Geometry check sheet. Reference: the model listing, model coordinates, mm. A direction names the side the tool comes from. Coordinates: 2 decimals unless noted, no trailing zeros. Loops run counter-clockwise (first coordinate to the right, second up) from the corner with the lowest first, then second, coordinate; pieces in that order, holes last.
Autodesk Inventor part; units mm, degrees
ref_plane "YZ Plane" through (0, 0, 0) normal (1, 0, 0) x (0, 1, 0)
ref_plane "XZ Plane" through (0, 0, 0) normal (0, 1, 0) x (-1, 0, 0)
ref_plane "XY Plane" through (0, 0, 0) normal (0, 0, 1) x (1, 0, 0)
sketch "スケッチ1" plane through (0, 0, 0) normal (0, 0, 1) x (1, 0, 0)
  line L0 (67.5, 17.5) -> (-67.5, 17.5) construction
  line L1 (-67.5, 17.5) -> (-67.5, -17.5) construction
  line L2 (-67.5, -17.5) -> (67.5, -17.5) construction
  line L3 (67.5, -17.5) -> (67.5, 17.5) construction
  line L4 (67.5, 17.5) -> (-67.5, -17.5) construction
  line L5 (-67.5, 17.5) -> (67.5, -17.5) construction
  circle A0 centre (-60, 35) radius 1.6 construction
  circle A1 centre (-70, 35) radius 1.6 construction
  line L6 (-77.5, 27.5) -> (-53, 27.5) construction
  line L7 (-53, 27.5) -> (-53, 42.5) construction
  line L8 (-53, 42.5) -> (-80, 42.5) construction
  line L9 (-77.5, 27.5) -> (-77.5, -27.5) construction
  line L10 (-77.5, -27.5) -> (-53, -27.5) construction
  line L11 (-53, -27.5) -> (-53, -42.5) construction
  line L12 (-53, -42.5) -> (-80, -42.5) construction
  circle A2 centre (-60, -35) radius 1.6 construction
  circle A3 centre (-70, -35) radius 1.6 construction
  circle A4 centre (-80, -35) radius 1.6 construction
  line L13 (124.2308, -31.7536) -> (484.5935, -392.1164)
  line L14 (484.5935, -392.1164) -> (488.7129, -553.575)
  line L15 (-80, 21.2868) -> (-468.838, -367.5512) construction
  line L16 (-468.838, -367.5512) -> (-479.4446, -356.9446)
  line L17 (-479.4446, -356.9446) -> (-90.6066, 31.8934) construction
  line L18 (-90.6066, 31.8934) -> (-80, 21.2868) construction
  line L19 (-80, 42.5) -> (-80, 5.3052) construction
  circle A5 centre (-92.3744, 19.519) radius 1.6 construction
  circle A6 centre (-102.981, 8.9124) radius 1.6 construction
  circle A7 centre (-113.5876, -1.6942) radius 1.6 construction
  line L20 (-92.3744, 19.519) -> (-113.5876, -1.6942) construction
  circle A8 centre (-437.941, -345.2067) radius 1.6
  circle A9 centre (-426.1402, -333.4059) radius 1.6
  line L21 (-388.4374, -772.2067) -> (-358.1265, -754.7067) construction
  line L22 (-358.1265, -754.7067) -> (-425.6265, -637.7933) construction
  line L23 (-455.9374, -655.2933) -> (-358.1265, -754.7067) construction
  line L24 (-388.4374, -772.2067) -> (-425.6265, -637.7933) construction
  line L25 (-455.9374, -655.2933) -> (-388.4374, -772.2067) construction
  line L26 (-425.6265, -637.7933) -> (-455.9374, -655.2933) construction
  line L27 (455.9374, -655.2933) -> (425.6265, -637.7933) construction
  line L28 (425.6265, -637.7933) -> (358.1265, -754.7067) construction
  line L29 (388.4374, -772.2067) -> (425.6265, -637.7933) construction
  line L30 (455.9374, -655.2933) -> (358.1265, -754.7067) construction
  line L31 (388.4374, -772.2067) -> (455.9374, -655.2933) construction
  line L32 (358.1265, -754.7067) -> (388.4374, -772.2067) construction
  line L33 (0, 0) -> (0, -263.4473) construction
  circle A10 centre (80, -35) radius 1.6 construction
  line L34 (67.5, 17.5) -> (67.5, -17.5) construction
  line L35 (77.5, 27.5) -> (53, 27.5) construction
  line L36 (77.5, 27.5) -> (77.5, -27.5) construction
  line L37 (77.5, -27.5) -> (53, -27.5) construction
  circle A11 centre (60, -35) radius 1.6 construction
  circle A12 centre (70, -35) radius 1.6 construction
  line L38 (53, -27.5) -> (53, -42.5) construction
  line L39 (53, -42.5) -> (80, -42.5) construction
  circle A13 centre (60, 35) radius 1.6 construction
  circle A14 centre (70, 35) radius 1.6 construction
  line L40 (80, 42.5) -> (80, 5.3052) construction
  line L41 (53, 42.5) -> (80, 42.5) construction
  line L42 (53, 27.5) -> (53, 42.5) construction
  line L43 (-392.0976, -785.867) -> (-404.3476, -764.6493)
  line L44 (-388.4374, -772.2067) -> (-358.1265, -754.7067) construction
  line L45 (-392.0976, -785.867) -> (-344.4662, -758.367)
  circle A15 centre (-336.7211, -756.782) radius 1.6
  circle A16 centre (-341.7211, -748.1218) radius 1.6
  line L46 (-343.7259, -729.6493) -> (-330.2259, -753.032)
  circle A17 centre (-346.7211, -739.4615) radius 1.6
  line L47 (-356.7162, -737.1493) -> (-343.7259, -729.6493)
  line L48 (-344.4662, -758.367) -> (-356.7162, -737.1493)
  circle A18 centre (-407.3428, -774.4615) radius 1.6
  circle A19 centre (-402.3428, -783.1218) radius 1.6
  line L49 (-404.3476, -764.6493) -> (-417.338, -772.1493)
  line L50 (-417.338, -772.1493) -> (-403.838, -795.532)
  line L51 (-403.838, -795.532) -> (-371.6264, -776.9346) construction
  line L52 (-425.6265, -637.7933) -> (-455.9374, -655.2933) construction
  line L53 (-409.7162, -645.3507) -> (-396.7259, -637.8507)
  circle A20 centre (-406.7211, -635.5385) radius 1.6
  line L54 (-455.9374, -655.2933) -> (-425.6265, -637.7933) construction
  circle A21 centre (-411.7211, -626.8782) radius 1.6
  line L55 (-469.5976, -651.633) -> (-421.9662, -624.133)
  line L56 (-421.9662, -624.133) -> (-409.7162, -645.3507)
  line L57 (-396.7259, -637.8507) -> (-410.2259, -614.468)
  circle A22 centre (-416.7211, -618.218) radius 1.6
  line L58 (-469.5976, -651.633) -> (-457.3476, -672.8507)
  circle A23 centre (-467.3428, -670.5385) radius 1.6
  circle A24 centre (-472.3428, -661.8782) radius 1.6
  line L59 (-483.838, -656.968) -> (-451.6264, -638.3706) construction
  line L60 (-470.338, -680.3507) -> (-483.838, -656.968)
  line L61 (-457.3476, -672.8507) -> (-470.338, -680.3507)
  line L62 (469.5976, -651.633) -> (457.3476, -672.8507)
  line L63 (455.9374, -655.2933) -> (425.6265, -637.7933) construction
  line L64 (469.5976, -651.633) -> (421.9662, -624.133)
  circle A25 centre (416.7211, -618.218) radius 1.6
  circle A26 centre (411.7211, -626.8782) radius 1.6
  line L65 (396.7259, -637.8507) -> (410.2259, -614.468)
  circle A27 centre (406.7211, -635.5385) radius 1.6
  line L66 (409.7162, -645.3507) -> (396.7259, -637.8507)
  line L67 (421.9662, -624.133) -> (409.7162, -645.3507)
  circle A28 centre (467.3428, -670.5385) radius 1.6
  circle A29 centre (472.3428, -661.8782) radius 1.6
  line L68 (457.3476, -672.8507) -> (470.338, -680.3507)
  line L69 (470.338, -680.3507) -> (483.838, -656.968)
  line L70 (483.838, -656.968) -> (451.6264, -638.3706) construction
  line L71 (358.1265, -754.7067) -> (388.4374, -772.2067) construction
  line L72 (356.7162, -737.1493) -> (343.7259, -729.6493)
  circle A30 centre (346.7211, -739.4615) radius 1.6
  line L73 (388.4374, -772.2067) -> (358.1265, -754.7067) construction
  circle A31 centre (341.7211, -748.1218) radius 1.6
  line L74 (392.0976, -785.867) -> (344.4662, -758.367)
  line L75 (344.4662, -758.367) -> (356.7162, -737.1493)
  line L76 (343.7259, -729.6493) -> (330.2259, -753.032)
  circle A32 centre (336.7211, -756.782) radius 1.6
  line L77 (392.0976, -785.867) -> (404.3476, -764.6493)
  circle A33 centre (407.3428, -774.4615) radius 1.6
  circle A34 centre (402.3428, -783.1218) radius 1.6
  line L78 (403.838, -795.532) -> (371.6264, -776.9346) construction
  line L79 (417.338, -772.1493) -> (403.838, -795.532)
  line L80 (404.3476, -764.6493) -> (417.338, -772.1493)
  line L81 (-483.838, -367.5512) -> (-468.838, -367.5512)
  line L82 (-468.838, -367.5512) -> (-468.838, -648.3077) construction
  line L83 (-468.838, -648.3077) -> (-483.838, -648.3077) construction
  line L84 (-483.838, -648.3077) -> (-483.838, -367.5512) construction
  line L85 (-283.2277, -604.4352) -> (-262.2277, -640.8083) construction
  line L86 (345.2492, -497.0108) -> (305.7786, -565.3759) construction
  line L87 (260.9224, -655.004) -> (-239.0776, -655.004) construction
  line L88 (-239.0776, -655.004) -> (-239.0776, -1155.004) construction
  line L89 (-239.0776, -1155.004) -> (260.9224, -1155.004) construction
  line L90 (260.9224, -1155.004) -> (260.9224, -655.004) construction
  line L91 (260.9224, -655.004) -> (-239.0776, -1155.004) construction
  line L92 (-239.0776, -655.004) -> (260.9224, -1155.004) construction
  line L93 (-12.841, -157.5) -> (15.1134, -157.5) construction
  circle A35 centre (-3.0548, -432.807) radius 212.5 construction
  line L94 (496.9452, 30.2659) -> (-503.0548, 30.2659) construction
  line L95 (-503.0548, 30.2659) -> (-503.0548, -969.7341) construction
  line L96 (-503.0548, -969.7341) -> (496.9452, -969.7341) construction
  line L97 (496.9452, -969.7341) -> (496.9452, 30.2659) construction
  line L98 (496.9452, 30.2659) -> (-503.0548, -969.7341) construction
  line L99 (-503.0548, 30.2659) -> (496.9452, -969.7341) construction
  circle A36 centre (-3.0548, -432.807) radius 250 construction
  line L100 (-80, 42.5) -> (-90.6066, 31.8934) construction
  line L101 (-80, 42.5) -> (-118.8909, 3.6091) construction
  line L102 (-118.8909, -6.2904) -> (-113.234, -11.9472) construction
  line L103 (-113.234, -11.9472) -> (-85.3433, -40.263) construction
  arc A37 (-118.8909, 3.6091) -> (-118.8909, -6.2904) centre (-113.9411, -1.3406) ccw construction
  arc A38 (-85.3433, -40.263) -> (-80, -42.5) centre (-80, -35) ccw construction
  line L104 (-80, 42.5) -> (-53, 42.5) construction
  circle A39 centre (-476.338, -638.3077) radius 1.6
  circle A40 centre (-476.338, -623.3077) radius 1.6
  circle A41 centre (-476.338, -608.3077) radius 1.6
  line L105 (-483.838, -656.968) -> (-483.838, -601.3077)
  line L106 (-483.838, -601.3077) -> (-468.838, -601.3077)
  line L107 (-468.838, -601.3077) -> (-415.4046, -610.8344)
  arc A42 (-410.2259, -614.468) -> (-415.4046, -610.8344) centre (-416.7211, -618.218) ccw
  point P0 (0, -470)
  point P1 (-102.981, 8.9124)
  point P2 (-77.5, 0)
  point P3 (-407.0319, -705)
  point P4 (-407.0319, -705)
  point P5 (407.0319, -705)
  point P6 (407.0319, -705)
  point P7 (77.5, 0)
  point P8 (-368.2819, -772.117)
  point P9 (-385.4668, -784.9254)
  point P10 (-445.7819, -637.883)
  point P11 (445.7819, -637.883)
  point P12 (465.4668, -646.3614)
  point P13 (368.2819, -772.117)
  point P14 (10.9224, -905.004)
  point P15 (-3.0548, -469.7341)
  point P16 (-123.8406, -1.3406)
  dimension "d4" = 135
  dimension "d5" = 35
  dimension "d6" = 3.2
  dimension "d7" = 3.2
  dimension "d8" = 10
  dimension "d9" = 15
  dimension "d10" = 10
  dimension "d11" = 7.5
  dimension "d12" = 7
  dimension "d13" = 70
  dimension "d14" = 3.2
  dimension "d15" = 3.2
  dimension "d16" = 3.2
  dimension "d17" = 10
  dimension "d18" = 10
  dimension "d19" = 7
  dimension "d20" = 15
  dimension "d21" = 7.5
  dimension "d22" = 10
  dimension "d23" = 10
  dimension "d24" = 135
  dimension "d25" = 15
  dimension "d26" = 10
  dimension "d27" = 3.2
  dimension "d28" = 3.2
  dimension "d29" = 3.2
  dimension "d30" = 10
  dimension "d31" = 15
  dimension "d32" = 15
  dimension "d33" = 7.5
  dimension "d34" = 45
  dimension "d35" = 3.2
  dimension "d36" = 3.2
  dimension "d37" = 360
  dimension "d38" = 360
  dimension "d39" = 470
  dimension "d40" = 15
  dimension "d41" = 200
  dimension "d42" = 200
  dimension "d43" = 500
  dimension "d44" = 500
  dimension "d45" = 200
  dimension "d46" = 425
  dimension "d47" = 1000
  dimension "d48" = 1000
  dimension "d49" = 42
  dimension "d50" = 500
  dimension "d51" = 7
  dimension "d52" = 7
  dimension "d53" = 3.2
  dimension "d54" = 3.2
  dimension "d55" = 3.2
  dimension "d56" = 15
  dimension "d57" = 15
  dimension "d58" = 7.5
  dimension "d59" = 10
  dimension "d60" = 7
extrude "押し出し1" add sketch "スケッチ1" along normal blind 3 contours L56 L55 L58 L61 L60 L105 L106 L107 A42 L57 L53
fillet "フィレット1" radius 7.5 3 edges at (-483.838, -601.3077, 1.5) (-468.838, -601.3077, 1.5) (-483.838, -656.968, 1.5)
fillet "フィレット2" radius 3 6 edges at (-470.338, -680.3507, 1.5) (-457.3476, -672.8507, 1.5) (-469.5976, -651.633, 1.5) (-421.9662, -624.133, 1.5) (-409.7162, -645.3507, 1.5) (-396.7259, -637.8507, 1.5)
sketch "スケッチ2" plane through (0, 0, 3) normal (0, 0, 1) x (1, 0, 0)
  line L0 (-468.838, -607.4023) -> (-468.838, -622.7758)
  line L1 (-468.838, -622.7758) -> (-428.0246, -614.679)
  line L2 (-428.0246, -614.679) -> (-468.838, -607.4023)
  line L3 (-468.838, -628.8928) -> (-468.838, -644.2663)
  line L4 (-468.838, -644.2663) -> (-428.2708, -620.8447)
  line L5 (-428.2708, -620.8447) -> (-468.838, -628.8928)
  line L6 (-415.4046, -610.8344) -> (-468.185, -601.4241)
  line L7 (-466.9996, -650.133) -> (-424.5643, -625.633)
  line L8 (-483.838, -608.8077) -> (-483.838, -654.9583)
  circle A0 centre (-416.7211, -618.218) radius 1.6 construction
  line L9 (-428.0246, -614.679) -> (-416.7211, -618.218) construction
  line L10 (-416.7211, -618.218) -> (-428.2708, -620.8447) construction
  point P0 (0, 0)
  dimension "d65" = 15
  dimension "d66" = 6
  dimension "d67" = 6
  dimension "d68" = 6
extrude "押し出し2" cut sketch "スケッチ2" against normal blind 10
fillet "フィレット3" radius 2 6 edges at (-468.838, -607.4023, 1.5) (-468.838, -622.7758, 1.5) (-428.0246, -614.679, 1.5) (-428.2708, -620.8447, 1.5) (-468.838, -628.8928, 1.5) (-468.838, -644.2663, 1.5)
properties part number "オムニ_前1" material "アルミニウム 6061"
(1) Access from +Z, -Z, +X, -X, +Y, -Y to the whole of each face (thin tool, end or side, straight path). Record for faces 1 (the cylindrical face through (-468.14, -608.27, 1.48)), 2 (the cylindrical face through (-458.557, -672.561, 1.521)).
Findings:
face 1: +Z, -Z
face 2: +Z, -Z, +X
(2) Sectioned sample at A-A on y = -633. Record the cut outline in (x, z), and give its area (3 significant figures).
Findings:
outline: (-483.84, 0) - (-468.84, 0) - (-468.84, 3) - (-483.84, 3) - close; (-449.32, 0) - (-437.32, 0) - (-437.32, 3) - (-449.32, 3) - close; (-416.85, 0) - (-399.53, 0) - (-399.53, 3) - (-416.85, 3) - close
area: 133 mm2
(3) Scan lines: L1, parallel to X at y = -637.5, z = 1.15; L2, parallel to Y at x = -441.5, z = 0.3; L3, parallel to Y at x = -460.5, z = 0.8. Record each from-to range of solid material in increasing order.
Findings:
L1: x = -483.84 to -477.72, -474.96 to -468.84, -457.12 to -445.12, -414.25 to -397.92
L2: y = -635.41 to -628.48, -623.47 to -617.35, -612.28 to -606.18
L3: y = -674.67 to -667.39, -646.38 to -639.45, -627.24 to -621.12, -608.89 to -602.79
(4) Sectioned sample at B-B on x = -443.5. Record the cut outline in (y, z), and give its area (3 significant figures).
Findings:
outline: (-636.57, 0) - (-629.64, 0) - (-629.64, 3) - (-636.57, 3) - close; (-623.87, 0) - (-617.75, 0) - (-617.75, 3) - (-623.87, 3) - close; (-611.92, 0) - (-605.83, 0) - (-605.83, 3) - (-611.92, 3) - close
area: 57.4 mm2
(5) Sectioned sample at C-C on z = 1.4. State how many separate pieces and enclosed holes the cut face has, and give its area (3 significant figures).
Findings:
separate pieces: 1
enclosed holes: 10
area: 2,500 mm2
(6) Gauge pin test, flat end, axial feed: pin 1 Ø1.5 at (y, z) = (-615, 2) entering from +X. Record the tip position at first contact, or that the pin passes through.
Findings:
pin 1: stops at x = -409.49
(7) Draft check along Y on faces 3 (the flat face through (-451, -640, 0)), 4 (the flat face through (-403.276, -641.632, 1.479)), 5 (the cylindrical face through (-467.81, -642.55, 1.48)). Enter one of: +Y half, -Y half, draft (parallel to the pull), parting line (faces both ways), or undercut.
Findings:
face 3: draft
face 4: -Y half
face 5: undercut
(8) Sectioned sample at D-D on y = -657.5. Record the cut outline in (x, z).
Findings:
outline: (-483.39, 0) - (-466.21, 0) - (-466.21, 3) - (-483.39, 3) - close
